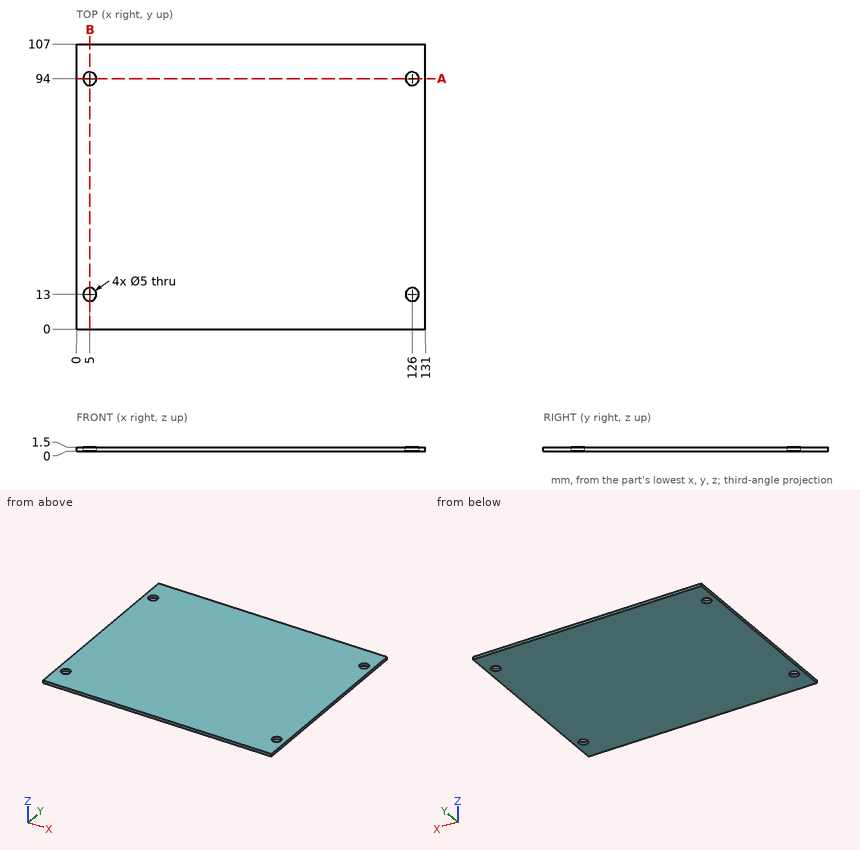
Print and shaded views of the part. All mm, measured from the part's lowest x, y and z. Give positions to 0.01 mm unless a question says otherwise; leave off trailing zeros. Loops run counter-clockwise (first coordinate to the right, second up) from the corner with the lowest first, then second, coordinate; pieces in that order, holes last. Notation, with made-up numbers: (-6.75, 12.5) -> (44.25, 12.5) arc R16 cw to (44.25, 40.5) -> close; hole circle Ø2 at (3, -28.5). An arc over 180 degrees is marked (long way). Use a Markdown table: item, result.
1. Slice it at B-B (x = 5). List the corners of the cut face in (y, z), plus the area to 4 significant figures.
Check result:
| item | result |
|---|---|
| outline | (0, 0) -> (10.5, 0) -> (10.5, 1.5) -> (0, 1.5) -> close; (15.5, 0) -> (91.5, 0) -> (91.5, 1.5) -> (15.5, 1.5) -> close; (96.5, 0) -> (107, 0) -> (107, 1.5) -> (96.5, 1.5) -> close |
| area | 145.5 mm^2 |
2. Wall check: L1, parallel to Y at x = 126, z = 1.1; L2, parallel to Y at x = 7, z = 0.1; L3, parallel to X at y = 94.5, z = 1.45. Give the ranges that are in metal, low to high. Write a range as [from, to].
Check result:
| item | result |
|---|---|
| L1 | y = [0, 10.5], [15.5, 91.5], [96.5, 107] |
| L2 | y = [0, 11.5], [14.5, 92.5], [95.5, 107] |
| L3 | x = [0, 2.55], [7.45, 123.55], [128.45, 131] |
3. Slice it at A-A (y = 94). List the corners of the cut face in (x, z), plus the area to 4 significant figures.
Check result:
| item | result |
|---|---|
| outline | (0, 0) -> (2.5, 0) -> (2.5, 1.5) -> (0, 1.5) -> close; (7.5, 0) -> (123.5, 0) -> (123.5, 1.5) -> (7.5, 1.5) -> close; (128.5, 0) -> (131, 0) -> (131, 1.5) -> (128.5, 1.5) -> close |
| area | 181.5 mm^2 |
